Could you check a few things on this drawing? It's one solid part, dimensions in mm from its lowest x, y, z. A direction names the side the tool comes from. Give positions to 0.01 mm unless a question says otherwise; leave off trailing zeros. Order: outer loops, then holes, each group sorted by start corner. A loop starts at its lowest first (then second) coordinate and runs counter-clockwise, first axis right, second up. Notation, with made-up numbers: (37, 67.25) -> (91, 67.25) arc R37 ccw to (91, 106.25) -> close; hole circle Ø4 at (-31.5, 13). An arc over 180 degrees is marked (long way). Answer as a JSON object with one key per item and string values.
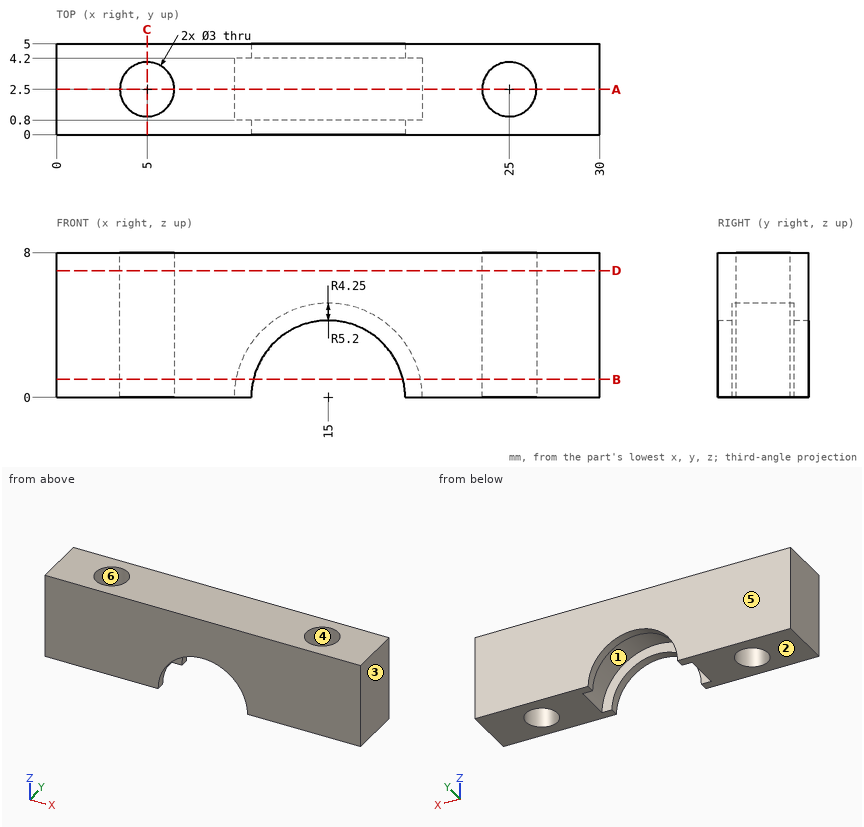
1. If we mould it in two halves opening along X, with no side actions, what happens to the marked faces 3, 4, 5 and 6? For each: +X half, -X half, draft (parallel to the pull), parting line (faces both ways), or undercut.
Worked answers:
{"face 3": "+X half", "face 4": "undercut", "face 5": "draft", "face 6": "undercut"}
2. Please list where these lines run through material, in increasing order: L1, parallel to X at y = 3.75, z = 0.5; L2, parallel to X at y = 3.65, z = 5.25; L3, parallel to X at y = 1.8, z = 1.
Worked answers:
{"L1": "0 to 4.17, 5.83 to 9.82, 20.18 to 24.17, 25.83 to 30", "L2": "0 to 4.04, 5.96 to 24.04, 25.96 to 30", "L3": "0 to 3.67, 6.33 to 9.9, 20.1 to 23.67, 26.33 to 30"}
3. If we section it at C-C on x = 5: Please give me the cut outline in (y, z), then the cut area to 3 significant figures.
Worked answers:
{"outline": "(0, 0) -> (1, 0) -> (1, 8) -> (0, 8) -> close; (4, 0) -> (5, 0) -> (5, 8) -> (4, 8) -> close", "area": "16.0 mm²"}
4. For the marked faces 1 and 2, which set-ups out of +Z, -Z, +X, -X, +Y, -Y let a thin tool reach every point of the face, with its end or its side?
Worked answers:
{"face 1": "-Z", "face 2": "-Z, +X, -X, +Y, -Y"}
5. Will this pin go through, and if not, where does the flat tip stop? pin 1 Ø1.6 at (x, z) = (14.5, 2.5) entering from +Y.
Worked answers:
{"pin 1": "through"}
6. If we section it at B-B on z = 1: Please give me the cut outline in (x, y).
Worked answers:
{"outline": "(0, 0) -> (10.87, 0) -> (10.87, 0.8) -> (9.9, 0.8) -> (9.9, 4.2) -> (10.87, 4.2) -> (10.87, 5) -> (0, 5) -> close; (19.13, 0) -> (30, 0) -> (30, 5) -> (19.13, 5) -> (19.13, 4.2) -> (20.1, 4.2) -> (20.1, 0.8) -> (19.13, 0.8) -> close; hole circle Ø3 at (5, 2.5); hole circle Ø3 at (25, 2.5)"}
7. If we section it at A-A on y = 2.5: Please give me the cut outline in (x, z).
Worked answers:
{"outline": "(0, 0) -> (3.5, 0) -> (3.5, 8) -> (0, 8) -> close; (6.5, 0) -> (9.8, 0) arc R5.2 cw to (20.2, 0) -> (23.5, 0) -> (23.5, 8) -> (6.5, 8) -> close; (26.5, 0) -> (30, 0) -> (30, 8) -> (26.5, 8) -> close"}
8. If we section it at D-D on z = 7: Please give me the cut outline in (x, y), then the cut area to 3 significant figures.
Worked answers:
{"outline": "(0, 0) -> (30, 0) -> (30, 5) -> (0, 5) -> close; hole circle Ø3 at (5, 2.5); hole circle Ø3 at (25, 2.5)", "area": "136 mm²"}
